The listing builds one solid part. Answer for the finished solid, in the listing's coordinates (mm). Face numbers are marked on the shaded views. A direction names the side the tool comes from. Give positions to 0.01 mm unless a question says otherwise; leave off trailing zeros. Loops run counter-clockwise (first coordinate to the right, second up) from the corner with the lowest first, then second, coordinate; pieces in that order, holes last. Notation, with made-up numbers: (-36.75, 53.25) - (-31.75, 53.25) arc R25 cw to (-31.75, 71.25) - close; hole circle Ø4 at (78, -25.75). An arc over 180 degrees is marked (long way). Write item = value, one per line. Start each with the question number.
1) The part is cut by section A-A on x = 0. Write down the section's boundary in (y, z), plus the area to 3 significant figures.
2) Which of the six approach directions +Z, -Z, +X, -X, +Y, -Y give full straight-line access (tool end or side, diameter ignored) to the marked faces 1 and 2?
3) The part is cut by section C-C on x = -8.25. Write down the section's boundary in (y, z), plus the area to 3 significant figures.
4) The part is cut by section D-D on y = -10.5. Write down the section's boundary in (x, z), plus the area to 3 significant figures.
5) Flat-ended cylindrical pins translate along their axes: P1, Ø4, axis at x = -6, y = 8, coming from the +Z side; P2, Ø1.5, axis at y = -5, z = 13, coming from the -X side; P3, Ø2, axis at x = 5, z = 13, coming from the -Y side; P4, Ø3.5, axis at x = -9.36, y = -9.36, coming from the -Z side. Find the tip coordinate at first contact, or state that the pin passes through.
6) Consider probe 1 along X at (y, z) = (-9.25, 1.5); probe 2 along X at (y, z) = (-8.5, 1). Determine where each line is inside the solid, lowest interval first.
7) The mould has two halves that part along X. Classify the marked faces 3, 4 and 5: +X half, -X half, draft (parallel to the pull), parting line (faces both ways), or undercut.
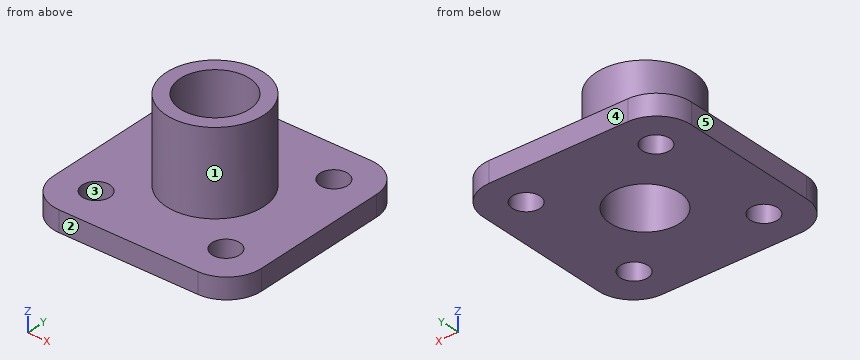
from build123d import *

# Parameters (mm, degrees)
F0_W     = 30
F0_H     = 30
F0_R     = 2
F0_R_2   = 7
F0_R_3   = 5
F1_DEPTH = 3
F2_DEPTH = 15
F3_R     = 5


with BuildPart() as f1:
    # F0 (on Top) → F1 (new body)
    with BuildSketch(Plane.XY):
        Rectangle(F0_W, F0_H)
        with Locations((-9.364547, -9.364547)):
            Circle(F0_R, mode=Mode.SUBTRACT)
        with Locations((9.364547, -9.364547)):
            Circle(F0_R, mode=Mode.SUBTRACT)
        with Locations((-9.364547, 9.364547)):
            Circle(F0_R, mode=Mode.SUBTRACT)
        Circle(F0_R_2, mode=Mode.SUBTRACT)
        with Locations((9.364547, 9.364547)):
            Circle(F0_R, mode=Mode.SUBTRACT)
        Circle(F0_R_2)
        Circle(F0_R_3, mode=Mode.SUBTRACT)
    extrude(amount=F1_DEPTH)

    # F0 (on Top) → F2 (join)
    with BuildSketch(Plane.XY):
        Circle(F0_R_2)
        Circle(F0_R_3, mode=Mode.SUBTRACT)
    extrude(amount=F2_DEPTH)

    # F3
    f3_edges = [f1.edges().sort_by_distance(p)[0] for p in [
        (-15, 15, 1.5),
        (15, 15, 1.5),
        (-15, -15, 1.5),
        (15, -15, 1.5),
    ]]
    fillet(f3_edges, radius=F3_R)


solid = f1.part
Answer below:
q1.outline = (-15, 0) - (-5, 0) - (-5, 15) - (-7, 15) - (-7, 3) - (-15, 3) - close; (5, 0) - (15, 0) - (15, 3) - (7, 3) - (7, 15) - (5, 15) - close
q1.area = 108 mm2
q2.face_1 = +Z
q2.face_2 = +Z, -Z, +X, -X, -Y
q3.outline = (-15, 0) - (-11.03, 0) - (-11.03, 3) - (-15, 3) - close; (-7.7, 0) - (7.7, 0) - (7.7, 3) - (-7.7, 3) - close; (11.03, 0) - (15, 0) - (15, 3) - (11.03, 3) - close
q3.area = 70.1 mm2
q4.outline = (-14.97, 0) - (-11.01, 0) - (-11.01, 3) - (-14.97, 3) - close; (-7.72, 0) - (7.72, 0) - (7.72, 3) - (-7.72, 3) - close; (11.01, 0) - (14.97, 0) - (14.97, 3) - (11.01, 3) - close
q4.area = 70.1 mm2
q5.P1 = 3
q5.P2 = -5.56
q5.P3 = -5.74
q5.P4 = through
q6.probe_1 = -15 to -11.36, -7.37 to 7.37, 11.36 to 15
q6.probe_2 = -15 to -11.17, -7.56 to 7.56, 11.17 to 15
q7.face_3 = undercut
q7.face_4 = draft
q7.face_5 = -X half
